Design review of the part built by this model. Coordinates are the model's own, in mm. Face numbers are marked on the shaded views. A direction names the side the tool comes from. Coordinates: 2 decimals unless noted, no trailing zeros. Write each loop counter-clockwise with the first axis right and the second up, starting at its lowest first coordinate (ties: lowest second). Pieces come first, ordered by that corner, then holes.
Q1. Take a section at B-B (y = 6.75). Give the boundary of the cut face in (x, z).
Q2. Take a section at A-A (x = 0). State how many separate pieces and enclosed holes the cut face has, and give its area (3 significant figures).
Q3. Insertion check: pin 1 (6 mm diameter, centred on x = -3, y = 10, fed in from -Z); pin 2 (1.6 mm diameter, centred on y = 2, z = -8.5, fed in from -X); pin 3 (1.9 mm diameter, centred on x = 0, z = 9, fed in from -Y); pin 4 (3 mm diameter, centred on x = -0.5, z = 8.5, fed in from +Y). Each pin has a flat end and moves straight along its axis. Give the tip position at first contact, or say it passes through.
Q4. Mouldability with a two-part tool opening along Z and no side actions: class the marked faces 1, 2 and 3 as pulls with the +Z half, pulls with the -Z half, needs draft (parallel to the pull), parting line crosses it, or undercut.
Q5. For probe 1 along Z at (x, y) = (0, 0.5); probe 2 along Z at (x, y) = (-4.5, 1); probe 3 along X at (y, z) = (1, 9), list the stretches that pass through material, from the lowest coordinate up.
Q6. Take a section at C-C (z = -3). Give the boundary of the cut face in (x, y), and give its area (3 significant figures).
Q7. Take a section at D-D (x = -6). Give the boundary of the cut face in (y, z).
Q8. Machinability: for the marked faces 4, 5 and 6, which of the approach directions +Z, -Z, +X, -X, +Y, -Y give a long, thin tool a straight path to every point of the face, cutting with its end or side? Answer none if there is none.
```python
from build123d import *

# Parameters (mm, degrees)
SKETCH1_W                = 11.6
SKETCH1_H                = 15
BODY_DEPTH               = 11.5
FLANGE_DEPTH             = 3
HOLDER_NUT_START         = 3
HOLDER_NUT_DEPTH         = 1.5
HOLE_M2_DEPTH            = 20.021960992
HOLE_M2_DEPTH_BACK       = 20.021960992
SKETCH8_R                = 1.2
FIXTURE_MOTOR_DEPTH      = 20.021960992
FIXTURE_MOTOR_DEPTH_BACK = 20.021960992
GEARBOX_NOTCHES_START    = -9.1
GEARBOX_NOTCHES_DEPTH    = 0.8


with BuildPart() as part:
    # Sketch1 → body (new body)
    with BuildSketch(Plane(origin=(0, 0, 0), x_dir=(1, 0, 0), z_dir=(0, 1, 0))):
        with Locations((-1.55, 0)):
            Rectangle(SKETCH1_W, SKETCH1_H)
    extrude(amount=BODY_DEPTH)

    # Sketch2 → flange (add)
    with BuildSketch(Plane(origin=(0, 0, 0), x_dir=(1, 0, 0), z_dir=(0, 1, 0))):
        with BuildLine():
            Line((-4.25, 9), (-4.25, 7.5))
            Line((-4.25, 7.5), (4.25, 7.5))
            Line((4.25, 7.5), (4.25, 9))
            ThreePointArc((4.25, 9), (0, 13.25), (-4.25, 9))
        make_face()
        with BuildLine():
            Line((4.25, -7.5), (4.25, -9))
            ThreePointArc((4.25, -9), (0, -13.25), (-4.25, -9))
            Line((-4.25, -9), (-4.25, -7.5))
            Line((-4.25, -7.5), (4.25, -7.5))
        make_face()
    extrude(amount=FLANGE_DEPTH)

    # Sketch5 → holder-nut (cut)
    with BuildSketch(Plane(origin=(0, 0, 0), x_dir=(1, 0, 0), z_dir=(0, 1, 0)).offset(HOLDER_NUT_START)):
        Polygon((2.25, 9), (1.125, 10.948557159), (-1.125, 10.948557159), (-2.25, 9), (-1.125, 7.051442841), (1.125, 7.051442841), align=None)
        Polygon((2.25, -9), (1.125, -7.051442841), (-1.125, -7.051442841), (-2.25, -9), (-1.125, -10.948557159), (1.125, -10.948557159), align=None)
    extrude(amount=-HOLDER_NUT_DEPTH, mode=Mode.SUBTRACT)

    # Sketch8 → hole-M2 (cut, two sides: drawn at the far end of the back side and taken through both)
    with BuildSketch(Plane(origin=(0, 0, 0), x_dir=(1, 0, 0), z_dir=(0, 1, 0)).offset(-HOLE_M2_DEPTH_BACK)):
        with Locations(Location((0, 9, 0), (0, 0, 270))):
            Circle(SKETCH8_R)
        with Locations(Location((0, -9, 0), (0, 0, 270))):
            Circle(SKETCH8_R)
    extrude(amount=HOLE_M2_DEPTH + HOLE_M2_DEPTH_BACK, mode=Mode.SUBTRACT)

    # Sketch7 → fixture-motor (cut, two sides: drawn at the far end of the back side and taken through both)
    with BuildSketch(Plane(origin=(0, 0, 0), x_dir=(0, 0, -1), z_dir=(1, 0, 0)).offset(-FIXTURE_MOTOR_DEPTH_BACK)):
        with BuildLine():
            Line((-4.5, 10), (4.5, 10))
            ThreePointArc((4.5, 10), (5.560660172, 9.560660172), (6, 8.5))
            Line((6, 8.5), (6, 0))
            Line((6, 0), (-6, 0))
            Line((-6, 0), (-6, 8.5))
            ThreePointArc((-6, 8.5), (-5.560660172, 9.560660172), (-4.5, 10))
        make_face()
    extrude(amount=FIXTURE_MOTOR_DEPTH + FIXTURE_MOTOR_DEPTH_BACK, mode=Mode.SUBTRACT)

    # Sketch9 → gearbox-notches (cut)
    with BuildSketch(Plane(origin=(4.25, 0, 0), x_dir=(0, 0, -1), z_dir=(1, 0, 0)).offset(GEARBOX_NOTCHES_START)):
        with BuildLine():
            Line((-6, 8.5), (-6, 10))
            Line((-6, 10), (-4.5, 10))
            ThreePointArc((-4.5, 10), (-5.560660172, 9.560660172), (-6, 8.5))
        make_face()
        with BuildLine():
            Line((4.5, 10), (6, 10))
            Line((6, 10), (6, 8.5))
            ThreePointArc((6, 8.5), (5.560660172, 9.560660172), (4.5, 10))
        make_face()
    extrude(amount=GEARBOX_NOTCHES_DEPTH, mode=Mode.SUBTRACT)


solid = part.part
```
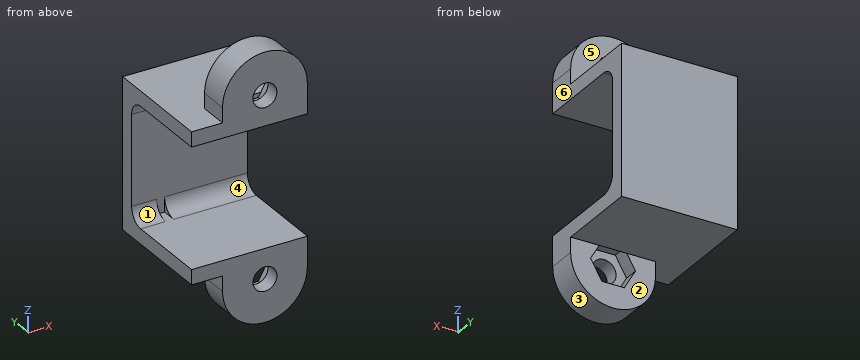
Response:
1. outline: (-7.35, -7.5) - (4.25, -7.5) - (4.25, -6) - (-7.35, -6) - close; (-7.35, 6) - (4.25, 6) - (4.25, 7.5) - (-7.35, 7.5) - close
2. separate pieces: 3
2. enclosed holes: 0
2. area: 69.1 mm2
3. pin 1: stops at z = -7.5
3. pin 2: stops at x = -4.25
3. pin 3: passes through
3. pin 4: stops at y = 11.5
4. face 1: undercut
4. face 2: needs draft
4. face 3: pulls with the -Z half
5. probe 1: z = -13.25 to -10.2, -7.8 to -6, 6 to 7.8, 10.2 to 13.25
5. probe 2: z = -7.5 to -6, 6 to 7.5
5. probe 3: x = -4.25 to -1.2, 1.2 to 4.25
6. outline: (-7.35, 10) - (4.25, 10) - (4.25, 11.5) - (-7.35, 11.5) - close
6. area: 17.4 mm2
7. outline: (0, -7.5) - (11.5, -7.5) - (11.5, 7.5) - (0, 7.5) - (0, 6) - (8.5, 6) arc R1.5 cw to (10, 4.5) - (10, -4.5) arc R1.5 cw to (8.5, -6) - (0, -6) - close
8. face 4: +X, -X, -Y
8. face 5: +Z, +X, -X, +Y
8. face 6: +Z, -Z, +X, +Y, -Y
